```python
from build123d import *

# Parameters (mm, degrees)
EXTRUDE_1_DEPTH        = 10
EXTRUDE_1_DEPTH_BACK   = 10
SKETCH_1_W             = 7
SKETCH_1_H             = 7
SKETCH_1_W_2           = 3.80020837
SKETCH_1_H_2           = 2.109580793
EXTRUDE_1_2_DEPTH      = 10
EXTRUDE_1_2_DEPTH_BACK = 10
SKETCH_2_W             = 5
SKETCH_2_H             = 3
SKETCH_2_R             = 0.977008115
EXTRUDE_2_DEPTH        = 7
EXTRUDE_3_REACH        = 22.928
FILLET_1_R             = 2
SKETCH_4_W             = 20
SKETCH_4_H             = 3
CUT_EXTRUDE_2_DEPTH    = 20


with BuildPart() as part:
    # Sketch 1 → Extrude 1 (new, two sides: drawn at the far end of the back side and taken through both)
    with BuildSketch(Plane(origin=(0, 0, 0), x_dir=(0, 0, -1), z_dir=(1, 0, 0)).offset(-EXTRUDE_1_DEPTH_BACK)):
        with Locations((-5, 3.5)):
            Rectangle(SKETCH_1_W, SKETCH_1_H)
        with Locations((-5, 4.821929683)):
            Rectangle(SKETCH_1_W_2, SKETCH_1_H_2, mode=Mode.SUBTRACT)
    extrude(amount=EXTRUDE_1_DEPTH + EXTRUDE_1_DEPTH_BACK)



with BuildPart() as body_2:
    # Sketch 1 → Extrude 1 2 (new, two sides: drawn at the far end of the back side and taken through both)
    with BuildSketch(Plane(origin=(0, 0, 0), x_dir=(0, 0, -1), z_dir=(1, 0, 0)).offset(-EXTRUDE_1_2_DEPTH_BACK)):
        with Locations((5, 3.5)):
            Rectangle(SKETCH_1_W, SKETCH_1_H)
        with Locations((5, 4.821929683)):
            Rectangle(SKETCH_1_W_2, SKETCH_1_H_2, mode=Mode.SUBTRACT)
    extrude(amount=EXTRUDE_1_2_DEPTH + EXTRUDE_1_2_DEPTH_BACK)


with BuildPart() as part_1:
    add(part.part)

    add(body_2.part)  # Extrude 2 merges body 2
    # Sketch 2 → Extrude 2 (add)
    with BuildSketch(Plane(origin=(0, 7, 0), x_dir=(1, 0, 0), z_dir=(0, 1, 0))):
        Rectangle(SKETCH_2_W, SKETCH_2_H)
        with Locations(Location((0, 0, 0), (0, 0, 270))):
            Circle(SKETCH_2_R, mode=Mode.SUBTRACT)
    extrude(amount=-EXTRUDE_2_DEPTH)

    # Extrude 3: up to this face of the body (flat: up to its plane)
    extrude_3_end = Plane(part_1.part.faces().sort_by_distance((0, 3.5, -8.5))[0])
    # Sketch 3 → Extrude 3 (add, up to the picked face)
    with BuildSketch(Plane.XY.offset(8.5), mode=Mode.PRIVATE) as extrude_3_sk1:
        with BuildLine():
            Line((-7.835690173, 14), (-7.835690173, 9.772160356))
            Line((-7.835690173, 9.772160356), (-3.020853064, 9.772160356))
            Line((-3.020853064, 9.772160356), (-3.020853064, 7))
            Line((-3.020853064, 7), (3.020853064, 7))
            Line((3.020853064, 7), (3.020853064, 9.772160356))
            Line((3.020853064, 9.772160356), (7.835690173, 9.772160356))
            Line((7.835690173, 9.772160356), (7.835690173, 14))
            ThreePointArc((7.835690173, 14), (0, 11.260367321), (-7.835690173, 14))
        make_face()
    extrude_3_tool1 = split(extrude(extrude_3_sk1.sketch, amount=-EXTRUDE_3_REACH, mode=Mode.PRIVATE), bisect_by=extrude_3_end, keep=Keep.BOTH, mode=Mode.PRIVATE)
    add(extrude_3_tool1.solids().sort_by(Axis((0, 10.244558, 8.5), (0, 0, -1)))[0])

    # Fillet 1
    fillet_1_edges = [part_1.edges().sort_by_distance(p)[0] for p in [
        (7.835690173, 14, 0),
        (-7.835690173, 14, 0),
    ]]
    fillet(fillet_1_edges, radius=FILLET_1_R)

    # Sketch 4 → Cut-Extrude 2 (cut)
    with BuildSketch(Plane(origin=(0, 7, 0), x_dir=(1, 0, 0), z_dir=(0, 1, 0))):
        Rectangle(SKETCH_4_W, SKETCH_4_H)
    extrude(amount=CUT_EXTRUDE_2_DEPTH, mode=Mode.SUBTRACT)


solid = part_1.part
```
Check sheet for the modelled part. Datum: model origin and axes. Units: mm. A direction names the side the tool comes from. Give positions to 0.01 mm unless a question says otherwise; leave off trailing zeros. Write each loop counter-clockwise with the first axis right and the second up, starting at its lowest first coordinate (ties: lowest second). Pieces come first, ordered by that corner, then holes.
Item 1: Access from +Z, -Z, +X, -X, +Y, -Y to the whole of each face (thin tool, end or side, straight path). Record for faces 5 (the face through (0, 8, -1.5)), 6 (the face through (-7, 7, -5)), 7 (the face through (0, 5.877, -5)), 8 (the face through (2.5, 4, 0)).
Item 2: Cross-section at D-D (y = 7.25). Enter the section's corners in (x, z).
Item 3: Cross-section at C-C (z = 0). Enter the section's corners in (x, y), and give its area (3 significant figures).
Item 4: Cross-section at B-B (y = 5.25). Enter the section's corners in (x, z), and give its area (3 significant figures).
Item 5: Gauge pin test, flat ends, axial feed: pin 1 (0.8 mm diameter, centred on y = 10, z = 5, fed in from +X); pin 2 (0.8 mm diameter, centred on y = 8, z = 3.5, fed in from -X); pin 3 (0.6 mm diameter, centred on y = 10, z = -6.5, fed in from -X); pin 4 (1.6 mm diameter, centred on x = 0, z = 0, fed in from +Y). Record the tip position at first contact, or that the pin passes through.
Item 6: Scan lines: L1, parallel to Z at x = 7.5, y = 4.5; L2, parallel to Y at x = -5.75, z = 7.75; L3, parallel to X at y = 5.25, z = 0. Record each from-to range of solid material in increasing order.
Item 7: Draft check along X on faces 1 (the face through (-3.021, 8, -5)), 2 (the face through (-0.867, 3.549, 0.451)), 3 (the face through (5, 9.772, 5)), 4 (the face through (10, 3.5, 5)). Enter one of: released by +X, released by -X, zero draft, split by the parting line, or undercut.
Item 8: Cross-section at A-A (x = 0). Enter the section's corners in (y, z), and give its area (3 significant figures).
Report:
1. face 5: +Y
1. face 6: +Z, -Z, -X
1. face 7: +X, -X
1. face 8: +X, +Y, -Y
2. outline: (-3.02, -8.5) - (3.02, -8.5) - (3.02, -1.5) - (-3.02, -1.5) - close; (-3.02, 1.5) - (3.02, 1.5) - (3.02, 8.5) - (-3.02, 8.5) - close
3. outline: (-2.5, 0) - (-0.98, 0) - (-0.98, 7) - (-2.5, 7) - close; (0.98, 0) - (2.5, 0) - (2.5, 7) - (0.98, 7) - close
3. area: 21.3 mm2
4. outline: (-10, -8.5) - (10, -8.5) - (10, -6.9) - (-10, -6.9) - close; (-10, -3.1) - (10, -3.1) - (10, -1.5) - (2.5, -1.5) - (2.5, 1.5) - (10, 1.5) - (10, 3.1) - (-10, 3.1) - (-10, 1.5) - (-2.5, 1.5) - (-2.5, -1.5) - (-10, -1.5) - close; (-10, 6.9) - (10, 6.9) - (10, 8.5) - (-10, 8.5) - close; hole circle Ø1.95 at (0, 0)
4. area: 140 mm2
5. pin 1: stops at x = 7.84
5. pin 2: stops at x = -3.02
5. pin 3: stops at x = -7.84
5. pin 4: passes through
6. L1: z = -8.5 to -6.9, -3.1 to -1.5, 1.5 to 3.1, 6.9 to 8.5
6. L2: y = 0 to 7, 9.77 to 12.48
6. L3: x = -2.5 to -0.98, 0.98 to 2.5
7. face 1: released by -X
7. face 2: undercut
7. face 3: zero draft
7. face 4: released by +X
8. outline: (0, -8.5) - (11.26, -8.5) - (11.26, -1.5) - (7, -1.5) - (7, -0.98) - (0, -0.98) - close; (0, 0.98) - (7, 0.98) - (7, 1.5) - (11.26, 1.5) - (11.26, 8.5) - (0, 8.5) - close; hole (3.77, -6.9) - (5.88, -6.9) - (5.88, -3.1) - (3.77, -3.1) - close; hole (3.77, 3.1) - (5.88, 3.1) - (5.88, 6.9) - (3.77, 6.9) - close
8. area: 149 mm2
